Source: CAD feature listing. Evaluate the final solid. Frame: model axes, mm. Round coordinates to 2 decimals unless told otherwise and drop trailing zeros. Loops run counter-clockwise (first coordinate to the right, second up) from the corner with the lowest first, then second, coordinate; pieces in that order, holes last. Notation, with made-up numbers: M 4.5,15.5 L 27.5,15.5 A16 ccw 27.5,19.5 Z; hole C 81.25,-36 d9. An arc over 180 degrees is marked long. Answer as a JSON object with one key per item and string values.
from build123d import *

# Parameters (mm, degrees)
F0_W      = 101.6
F0_H      = 101.6
F1_DEPTH  = 50.8
F6_W      = 98.9533215761
F6_H      = 109.5847634133
F7_DEPTH  = 29.3303936748
F9_R      = 55.4258032392
F10_DEPTH = 29.3303936748
F12_R     = 66.861305092
F13_DEPTH = 29.3303936748
F15_R     = 63.7455085669
F16_DEPTH = 29.3303936748
F21_R     = 117.7935216741
F22_DEPTH = 29.3303936748
F24_R     = 77.2031317043
F25_DEPTH = 29.3303936748
F27_R     = 77.6037163902
F28_DEPTH = 29.3303936748
F30_R     = 68.124609224
F31_DEPTH = 29.3303936748
F32_R     = 25.4
F33_DEPTH = 101.601
F34_R     = 25.4
F35_DEPTH = 101.601
F36_R     = 25.4
F37_DEPTH = 101.601


with BuildPart() as f1:
    # F0 (on Top) → F1 (new body, symmetric)
    with BuildSketch(Plane.XY):
        Rectangle(F0_W, F0_H)
    extrude(amount=F1_DEPTH, both=True)

    # F6 (on face) → F7 (cut, through all)
    with BuildSketch(Plane(origin=(-33.8666666667, -33.8666666667, 33.8666666667), x_dir=(0.8164965809, -0.4082482905, 0.4082482905), z_dir=(-0.5773502692, -0.5773502692, 0.5773502692))):
        with Locations((0, -1.2222639052)):
            Rectangle(F6_W, F6_H)
    extrude(amount=F7_DEPTH, mode=Mode.SUBTRACT)

    # F9 (on face) → F10 (cut, through all)
    with BuildSketch(Plane(origin=(33.8666666667, -33.8666666667, 33.8666666667), x_dir=(0.8164965809, 0.4082482905, -0.4082482905), z_dir=(-0.5773502692, 0.5773502692, -0.5773502692))):
        with Locations((-7.7910861, -7.1166269481)):
            Circle(F9_R)
    extrude(amount=-F10_DEPTH, mode=Mode.SUBTRACT)

    # F12 (on face) → F13 (cut, through all)
    with BuildSketch(Plane(origin=(-33.8666666667, 33.8666666667, 33.8666666667), x_dir=(0.8164965809, 0.4082482905, 0.4082482905), z_dir=(0.5773502692, -0.5773502692, -0.5773502692))):
        with Locations((-13.3071886376, -3.545607673)):
            Circle(F12_R)
    extrude(amount=-F13_DEPTH, mode=Mode.SUBTRACT)

    # F15 (on face) → F16 (cut, through all)
    with BuildSketch(Plane(origin=(-33.8666666667, -33.8666666667, -33.8666666667), x_dir=(0.8164965809, -0.4082482905, -0.4082482905), z_dir=(-0.5773502692, -0.5773502692, -0.5773502692))):
        with Locations((-3.3120266162, -3.843720071)):
            Circle(F15_R)
    extrude(amount=F16_DEPTH, mode=Mode.SUBTRACT)

    # F21 (on face) → F22 (cut, through all)
    with BuildSketch(Plane(origin=(33.8666666667, 33.8666666667, 33.8666666667), x_dir=(0.8164965809, -0.4082482905, -0.4082482905), z_dir=(-0.5773502692, -0.5773502692, -0.5773502692))):
        with Locations((0, -4.4537498616)):
            Circle(F21_R)
    extrude(amount=-F22_DEPTH, mode=Mode.SUBTRACT)

    # F24 (on face) → F25 (cut, through all)
    with BuildSketch(Plane(origin=(33.8666666667, 33.8666666667, -33.8666666667), x_dir=(-0.4082482905, 0.8164965809, 0.4082482905), z_dir=(0.5773502692, 0.5773502692, -0.5773502692))):
        with Locations((-11.0818976536, -8.1726238132)):
            Circle(F24_R)
    extrude(amount=F25_DEPTH, mode=Mode.SUBTRACT)

    # F27 (on face) → F28 (cut, through all)
    with BuildSketch(Plane(origin=(33.8666666667, -33.8666666667, -33.8666666667), x_dir=(-0.8164965809, -0.4082482905, -0.4082482905), z_dir=(-0.5773502692, 0.5773502692, 0.5773502692))):
        with Locations((0, -3.7476688158)):
            Circle(F27_R)
    extrude(amount=-F28_DEPTH, mode=Mode.SUBTRACT)

    # F30 (on face) → F31 (cut, through all)
    with BuildSketch(Plane(origin=(-33.8666666667, 33.8666666667, -33.8666666667), x_dir=(0.4082482905, 0.8164965809, 0.4082482905), z_dir=(0.5773502692, -0.5773502692, 0.5773502692))):
        with Locations((-6.1401822604, -7.8550539911)):
            Circle(F30_R)
    extrude(amount=-F31_DEPTH, mode=Mode.SUBTRACT)

    # F32 (on face) → F33 (cut, through all)
    with BuildSketch(Plane.XY.offset(50.8)):
        with Locations((1.4577903733, 0)):
            Circle(F32_R)
    extrude(amount=-F33_DEPTH, mode=Mode.SUBTRACT)

    # F34 (on face) → F35 (cut, through all)
    with BuildSketch(Plane.XZ.offset(50.8)):
        Circle(F34_R)
    extrude(amount=-F35_DEPTH, mode=Mode.SUBTRACT)

    # F36 (on face) → F37 (cut, through all)
    with BuildSketch(Plane.YZ.offset(50.8)):
        Circle(F36_R)
    extrude(amount=-F37_DEPTH, mode=Mode.SUBTRACT)


solid = f1.part
Item 1: Contact query for flat-ended pins moving along their axis: pin 1 Ø5 at (x, z) = (-22.5, 35.5) entering from +Y; pin 2 Ø12 at (x, y) = (19, -37) entering from -Z. Output: stop coordinate, or through.
Answer sheet:
{"pin 1": "stops at y = 47.14", "pin 2": "stops at z = -50.8"}
Item 2: Section D-D on x = -34.5. Return the cut outline in (y, z).
Answer sheet:
{"outline": "M -50.8,-16.3 L -16.3,-50.8 L 16.3,-50.8 L 50.8,-16.3 L 50.8,16.3 L 16.3,50.8 L -16.3,50.8 L -50.8,16.3 Z; hole C 0,0 d50.8"}
Item 3: Line query: probe 1 along Z at (x, y) = (0, -36); probe 2 along Y at (x, z) = (0.5, 40); probe 3 along X at (y, z) = (0, -29). Output: solid intervals per line, ascending. Write a range as from..to.
Answer sheet:
{"probe 1": "z = -50.8..-25.4, 25.4..50.8", "probe 2": "y = -50.8..-25.38, 25.38..50.8", "probe 3": "x = -50.8..-23.94, 26.86..50.8"}
Item 4: Section C-C on z = -20.5. Return the cut outline in (x, y).
Answer sheet:
{"outline": "M -50.8,-30.3 L -30.3,-50.8 L -15,-50.8 L -15,-19.35 A25.4 cw -19.04,-15 L -50.8,-15 Z; M -50.8,15 L -19.04,15 A25.4 cw -15,19.35 L -15,50.8 L -30.3,50.8 L -50.8,30.3 Z; M 15,-50.8 L 30.3,-50.8 L 50.8,-30.3 L 50.8,-15 L 21.96,-15 A25.4 cw 15,-21.49 Z; M 15,21.49 A25.4 cw 21.96,15 L 50.8,15 L 50.8,30.3 L 30.3,50.8 L 15,50.8 Z"}
Item 5: Section B-B on x = -12. Return the cut outline in (y, z), then the cut area to 3 significant figures.
Answer sheet:
{"outline": "M -50.8,-38.8 L -38.8,-50.8 L -21.54,-50.8 L -21.54,-22.39 L -50.8,-22.39 Z; M -50.8,22.39 L -21.54,22.39 L -21.54,50.8 L -38.8,50.8 L -50.8,38.8 Z; M 21.54,-50.8 L 38.8,-50.8 L 50.8,-38.8 L 50.8,-22.39 L 21.54,-22.39 Z; M 21.54,22.39 L 50.8,22.39 L 50.8,38.8 L 38.8,50.8 L 21.54,50.8 Z", "area": "3,040 mm²"}
Item 6: Pull-direction query (Y, two-part tool) for faces 1 (the flat face through (0, 50.8, -26)), 2 (the cylindrical face through (-17.26, 17.17, 37.97)), 3 (the flat face through (-50.8, 0, -26)); classes: pulls with the +Y half, pulls with the -Y half, needs draft (parallel to the pull), parting line crosses it, or undercut.
Answer sheet:
{"face 1": "pulls with the +Y half", "face 2": "undercut", "face 3": "needs draft"}
Item 7: Section A-A on y = -35. Return the cut outline in (x, z), then the cut area to 3 significant figures.
Answer sheet:
{"outline": "M -50.8,-15.8 L -15.8,-50.8 L 15.8,-50.8 L 50.8,-15.8 L 50.8,15.8 L 15.8,50.8 L -15.8,50.8 L -50.8,15.8 Z; hole C 0,0 d50.8", "area": "5,850 mm²"}
